```python
from build123d import *

# Parameters (mm, degrees)
EXTRUDE_1_DEPTH     = 225
SHELL_2_T           = 2.5
SKETCH_2_R          = 2.5
CUT_EXTRUDE_1_DEPTH = 236.239239924


with BuildPart() as part:
    # 草图1 → 凸台-拉伸1 (new body)
    with BuildSketch(Plane.XY):
        with BuildLine():
            Line((-39, 17.5), (39, 17.5))
            ThreePointArc((39, 17.5), (50.313708499, 12.813708499), (55, 1.5))
            Line((55, 1.5), (55, -17.5))
            Line((55, -17.5), (-55, -17.5))
            Line((-55, -17.5), (-55, 1.5))
            ThreePointArc((-55, 1.5), (-50.313708499, 12.813708499), (-39, 17.5))
        make_face()
    extrude(amount=EXTRUDE_1_DEPTH)

    # 抽壳2
    shell_2_openings = [part.faces().sort_by_distance(p)[0] for p in [
        (0, -17.5, 112.5),
        (0, -0.40911681, 0),
        (0, -0.40911681, 225),
    ]]
    offset(amount=SHELL_2_T, openings=shell_2_openings, kind=Kind.INTERSECTION)

    # 草图2 → 切除-拉伸1 (cut, through all)
    with BuildSketch(Plane(origin=(0, 20, 0), x_dir=(1, 0, 0), z_dir=(0, 1, 0))):
        with Locations(Location((-12, -7.5, 0), (0, 0, 270))):
            Circle(SKETCH_2_R)
        with Locations(Location((12, -7.5, 0), (0, 0, 270))):
            Circle(SKETCH_2_R)
        with Locations(Location((-12, -217.5, 0), (0, 0, 90))):
            Circle(SKETCH_2_R)
        with Locations(Location((12, -217.5, 0), (0, 0, 90))):
            Circle(SKETCH_2_R)
        with BuildLine():
            Line((-14, 0), (-74.033168475, 0))
            Line((-74.033168475, 0), (-74.033168475, -15))
            Line((-74.033168475, -15), (-57.5, -15))
            Line((-57.5, -15), (-22, -15))
            ThreePointArc((-22, -15), (-19.171572875, -13.828427125), (-18, -11))
            Line((-18, -11), (-18, -4))
            ThreePointArc((-18, -4), (-16.828427125, -1.171572875), (-14, 0))
        make_face()
        with BuildLine():
            Line((57.5, -15), (57.5, 0))
            Line((57.5, 0), (14, 0))
            ThreePointArc((14, 0), (16.828427125, -1.171572875), (18, -4))
            Line((18, -4), (18, -11))
            ThreePointArc((18, -11), (19.171572875, -13.828427125), (22, -15))
            Line((22, -15), (57.5, -15))
        make_face()
        with BuildLine():
            Line((18, -221), (18, -214))
            ThreePointArc((18, -214), (19.171572875, -211.171572875), (22, -210))
            Line((22, -210), (57.5, -210))
            Line((57.5, -210), (57.5, -225))
            Line((57.5, -225), (14, -225))
            ThreePointArc((14, -225), (16.828427125, -223.828427125), (18, -221))
        make_face()
        with BuildLine():
            Line((-18, -221), (-18, -214))
            ThreePointArc((-18, -214), (-19.171572875, -211.171572875), (-22, -210))
            Line((-22, -210), (-57.5, -210))
            Line((-57.5, -210), (-74.033168475, -210))
            Line((-74.033168475, -210), (-74.033168475, -225))
            Line((-74.033168475, -225), (-14, -225))
            ThreePointArc((-14, -225), (-16.828427125, -223.828427125), (-18, -221))
        make_face()
    extrude(amount=-CUT_EXTRUDE_1_DEPTH, mode=Mode.SUBTRACT)


solid = part.part
```
Geometry check sheet. Reference: the model listing, model coordinates, mm. A direction names the side the tool comes from. Round coordinates to 2 decimals unless told otherwise and drop trailing zeros. Order: outer loops, then holes, each group sorted by start corner. A loop starts at its lowest first (then second) coordinate and runs counter-clockwise, first axis right, second up. Notation, with made-up numbers: M -10.5,-39 L 21.5,-39 A12 ccw 21.5,-28 Z; hole C 87.5,49.25 d11. An arc over 180 degrees is marked long. Answer as CSV lines item,"result".
1) Thickness scan on probe 1 along X at (y, z) = (18.2, 7.5); probe 2 along X at (y, z) = (18, 217); probe 3 along X at (y, z) = (-13, 152). Record the ranges inside material, lowest first. Write a range as [from, to].
Entries:
probe 1,"[-18, -14.5], [-9.5, 9.5], [14.5, 18]"
probe 2,"[-18, -14.45], [-9.55, 9.55], [14.45, 18]"
probe 3,"[-57.5, -55], [55, 57.5]"
2) Sectioned sample at A-A on z = 217.5. Record the cut outline in (x, y), and give its area (3 significant figures).
Entries:
outline,"M -18,17.5 L -14.5,17.5 L -14.5,20 L -18,20 Z; M -9.5,17.5 L 9.5,17.5 L 9.5,20 L -9.5,20 Z; M 14.5,17.5 L 18,17.5 L 18,20 L 14.5,20 Z"
area,"65.0 mm2"
3) Tool access check on faces 4 (the face through (53, 10, 15)), 5 (the face through (-50.437, 12.689, 111.135)), 6 (the face through (53, 10, 210)). Record the directions out of +Z, -Z, +X, -X, +Y, -Y that give a thin tool (end or side, any length) a straight path to the whole face; none if there is none.
Entries:
face 4,"-Z, +X, +Y, -Y"
face 5,"+Z, -Z, -Y"
face 6,"+Z, +X, +Y, -Y"
4) Mould release check, pull along Z, two halves, no side actions. Record for faces 1 (the face through (19.141, 18.768, 211.203)), 2 (the face through (-52.22, 14.44, 111.14)), 3 (the face through (12.96, 18.77, 215.19)): +Z half, -Z half, draft (parallel to the pull), parting line (faces both ways), or undercut.
Entries:
face 1,"+Z half"
face 2,"draft"
face 3,"undercut"
5) Sectioned sample at C-C on z = 141. Record the cut outline in (x, y), and give its area (3 significant figures).
Entries:
outline,"M -57.5,-17.5 L -55,-17.5 L -55,1.5 A16 cw -39,17.5 L 39,17.5 A16 cw 55,1.5 L 55,-17.5 L 57.5,-17.5 L 57.5,1.5 A18.5 ccw 39,20 L -39,20 A18.5 ccw -57.5,1.5 Z"
area,"425 mm2"
6) Sectioned sample at B-B on y = 12.5. Record the cut outline in (x, z), and give its area (3 significant figures).
Entries:
outline,"M -53.87,15 L -50.62,15 L -50.62,210 L -53.87,210 Z; M 50.62,15 L 53.87,15 L 53.87,210 L 50.62,210 Z"
area,"1,270 mm2"
7) Gauge pin test, flat ends, axial feed: pin 1 Ø8 at (x, y) = (-44, 8) entering from -Z; pin 2 Ø8 at (x, z) = (12, 7.5) entering from +Y; pin 3 Ø0.8 at (y, z) = (18.5, 9) entering from -X; pin 4 Ø0.8 at (y, z) = (18.5, 216) entering from +X. Record the tip position at first contact, or that the pin passes through.
Entries:
pin 1,"through"
pin 2,"y = 20"
pin 3,"x = -18"
pin 4,"x = 18"
8) Sectioned sample at D-D on y = -1.5. Record the cut outline in (x, z).
Entries:
outline,"M -57.5,15 L -55,15 L -55,210 L -57.5,210 Z; M 55,15 L 57.5,15 L 57.5,210 L 55,210 Z"
